Geometry: see drawing. Coordinates: mm, zero at the bounding-box minimum. Give positions to 0.01 mm unless a question says otherwise; leave off trailing zeros. Order: outer loops, then holes, each group sorted by start corner. A loop starts at its lowest first (then second) coordinate and runs counter-clockwise, first axis right, second up. Notation, with made-up numbers: M -25.75,-4 L -8.75,-4 A28 ccw -8.75,23 Z; hole C -30,26 d3. An arc over 180 degrees is marked long. Write item = value, one per line. Start each with the question number.
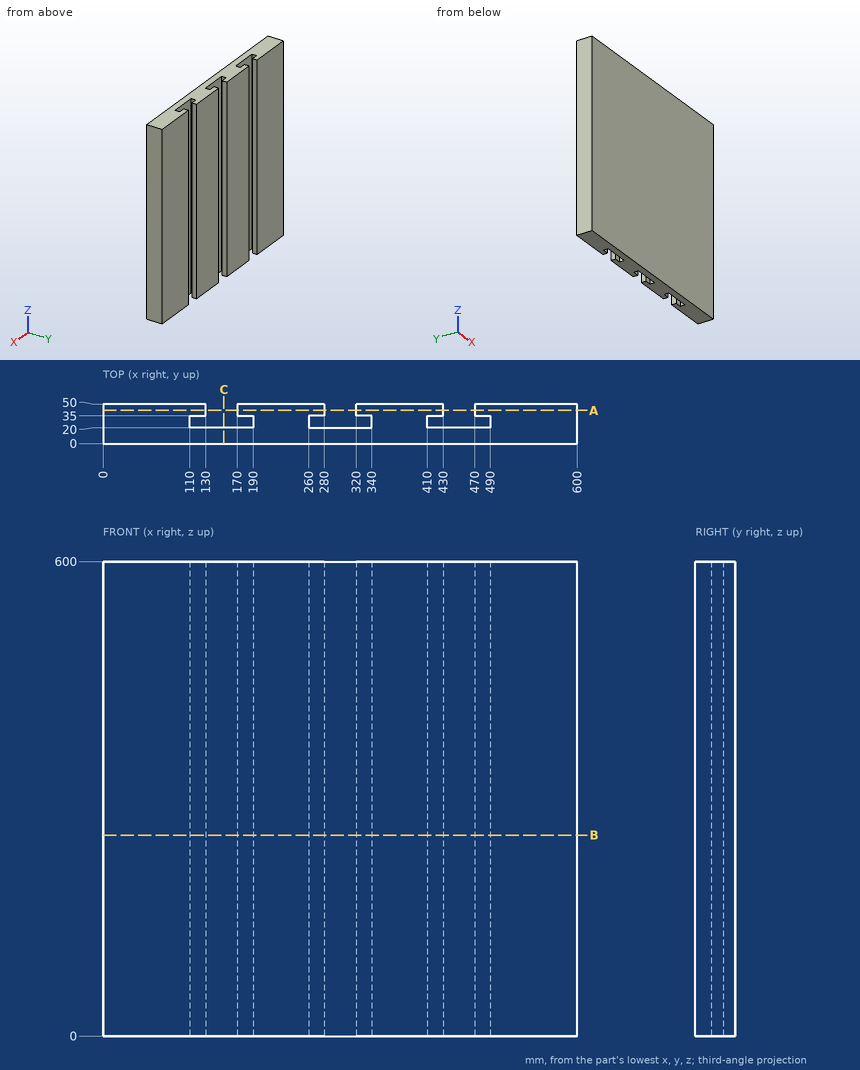
1) Cut plane B-B (z = 254). Return loops of the section in (x, y).
2) Cut plane C-C (x = 153). Return loops of the section in (y, z).
3) Pin query (flat end, axial travel): pin 1 Ø24 at (x, z) = (455.5, 262) entering from +Y. Return the tip coordinate at first contact, or that it passes through.
4) Ray query, L1, parallel to X at y = 36, z = 304; L2, parallel to X at y = 27.5, z = 360; L3, parallel to Y at x = 261, z = 62. Return the intervals inside material, ascending.
5) Cut plane A-A (y = 42). Return loops of the section in (x, z).
Reply:
q1.outline = M 0,0 L 600,0 L 600,50 L 470,50 L 470,35 L 490,35 L 490,20 L 410,20 L 410,35 L 430,35 L 430,50 L 320,50 L 320,35 L 340,35 L 340,20 L 260,20 L 260,35 L 280,35 L 280,50 L 170,50 L 170,35 L 190,35 L 190,20 L 110,20 L 110,35 L 130,35 L 130,50 L 0,50 Z
q2.outline = M 0,0 L 20,0 L 20,600 L 0,600 Z
q3.pin_1 = 20
q4.L1 = 0 to 130, 170 to 280, 320 to 430, 470 to 600
q4.L2 = 0 to 110, 190 to 260, 340 to 410, 490 to 600
q4.L3 = 0 to 20, 35 to 50
q5.outline = M 0,0 L 130,0 L 130,600 L 0,600 Z; M 170,0 L 280,0 L 280,600 L 170,600 Z; M 320,0 L 430,0 L 430,600 L 320,600 Z; M 470,0 L 600,0 L 600,600 L 470,600 Z
